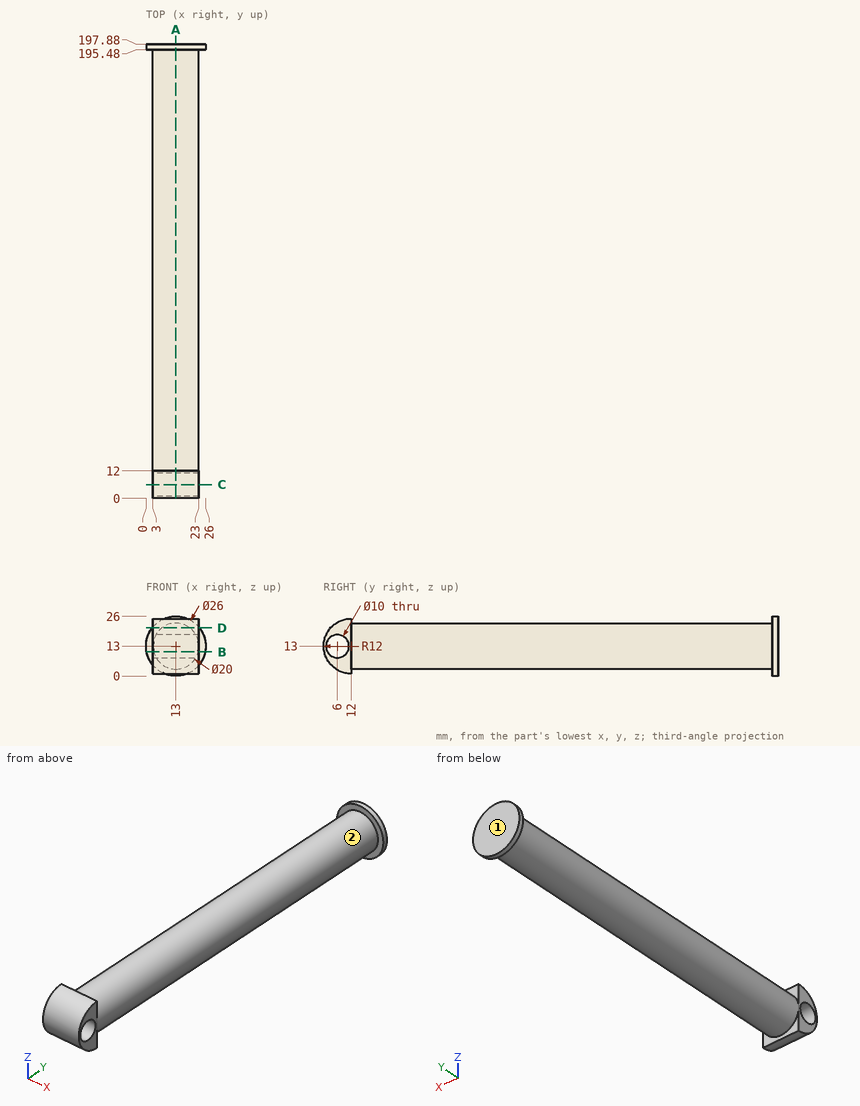
Answer from the drawing. Dimensions are ordinates in mm from the lowest x, y and z of the part. A direction names the side the tool comes from. Coordinates: 2 decimals unless noted, no trailing zeros. Write each loop counter-clockwise with the first axis right and the second up, starting at its lowest first coordinate (ties: lowest second). Pieces come first, ordered by that corner, then holes. Notation, with made-up numbers: M 34.5,-12.5 L 66.5,-12.5 A30 ccw 66.5,25.5 Z; hole C 89,-25.5 d6. An arc over 180 degrees is marked long. Write item = value, one per line.
1. Straight lines are drawn through the part: line 1 (Y direction, x = 15.75, z = 13); line 2 (Y direction, x = 21.25, z = 10.5); line 3 (X direction, y = 10, z = 9.5). For each, find the intervals that lie inside material, in ascending order. Write a range as from..to.
Solution:
line_1 = 0..1, 11..197.88
line_2 = 0.26..1.67, 10.33..197.88
line_3 = 3..23
2. The part is cut by section C-C (y = 6). Determine the outline of the cut face in (x, z), then the cut area to 3 significant figures.
Solution:
outline = M 3,2.61 L 23,2.61 L 23,8 L 3,8 Z; M 3,18 L 23,18 L 23,23.39 L 3,23.39 Z
area = 216 mm2
3. The part is cut by section A-A (x = 13). Determine the outline of the cut face in (y, z), then the cut area to 3 significant figures.
Solution:
outline = M 12,1 L 12,3 L 195.48,3 L 195.48,0 L 197.88,0 L 197.88,26 L 195.48,26 L 195.48,23 L 12,23 L 12,25 A12 ccw Z; hole C 6,13 d10
area = 3,880 mm2
4. For the marked faces 1 and 2, determine the directions among +Z, -Z, +X, -X, +Y, -Y from which every point of the face is accessible in a straight line to the end or side of a thin tool.
Solution:
face_1 = +Z, -Z, +X, -X, +Y
face_2 = none
5. Flat-ended cylindrical pins translate along their axes: pin 1 (6 mm diameter, centred on y = 4, z = 15.5, fed in from -X); pin 2 (8 mm diameter, centred on x = 11, y = 86.5, fed in from +Z); pin 3 (12 mm diameter, centred on x = 21.5, y = 152, fed in from +Z). Find the tip coordinate at first contact, or state that the pin passes through.
Solution:
pin_1 = 3
pin_2 = 23
pin_3 = 22.68
6. The part is cut by section B-B (z = 10.5). Determine the outline of the cut face in (x, y), then the cut area to 3 significant figures.
Solution:
outline = M 0.24,195.48 L 3.32,195.48 L 3.32,12 L 3,12 L 3,10.33 L 23,10.33 L 23,12 L 22.68,12 L 22.68,195.48 L 25.76,195.48 L 25.76,197.88 L 0.24,197.88 Z; M 3,0.26 L 23,0.26 L 23,1.67 L 3,1.67 Z
area = 3,680 mm2
7. The part is cut by section D-D (z = 21). Determine the outline of the cut face in (x, y), then the cut area to 3 significant figures.
Solution:
outline = M 2.75,195.48 L 7,195.48 L 7,12 L 3,12 L 3,3.06 L 23,3.06 L 23,12 L 19,12 L 19,195.48 L 23.25,195.48 L 23.25,197.88 L 2.75,197.88 Z
area = 2,430 mm2
